Drawing for the job (mm, zero at the part's lowest x, y, z). A direction names the side the tool comes from. Give positions to 0.01 mm unless a question says otherwise; leave off trailing zeros. Loops run counter-clockwise (first coordinate to the right, second up) from the corner with the lowest first, then second, coordinate; pieces in that order, holes last. Notation, with made-up numbers: (36.25, -36) -> (43.25, -36) arc R16 ccw to (43.25, -6) -> close; hole circle Ø10 at (45, -6.5). An arc over 180 degrees is marked (long way). Use CSV: the item, a comma, the result in double quotes. Start each with the question number.
(1) Cut at D-D on z = 9. Write the cut outline in (x, y).
(2) Cut at B-B on y = 26.25. State how many separate pieces and enclosed holes the cut face has, then the cut area to 3 significant figures.
(3) 3-axis set-ups, long thin cutter, end or side, ignore diameter. For the marked faces 1, 2, 3, 4 and 5: which of +Z, -Z, +X, -X, +Y, -Y reach the whole face in a straight line?
(4) Drill centre lines: probe 1 along X at (y, z) = (26.8, 3); probe 2 along Z at (x, y) = (41.7, 19); probe 3 along Y at (x, z) = (7, 26.5). Where is each one in solid material? Low to high.
(5) Cut at C-C on x = 27. Write the cut outline in (y, z), then the cut area to 3 significant figures.
(6) Flat gauge pins, fed straight in: pin 1 (2.5 mm diameter, centred on y = 16.5, z = 8.5, fed in from -X); pin 2 (2 mm diameter, centred on x = 43, y = 10, fed in from -Z); pin 3 (2.5 mm diameter, centred on x = 37, y = 8, fed in from +Z). Where does each tip first touch, or does it go through?
(7) Cut at A-A on z = 15. Write the cut outline in (x, y).
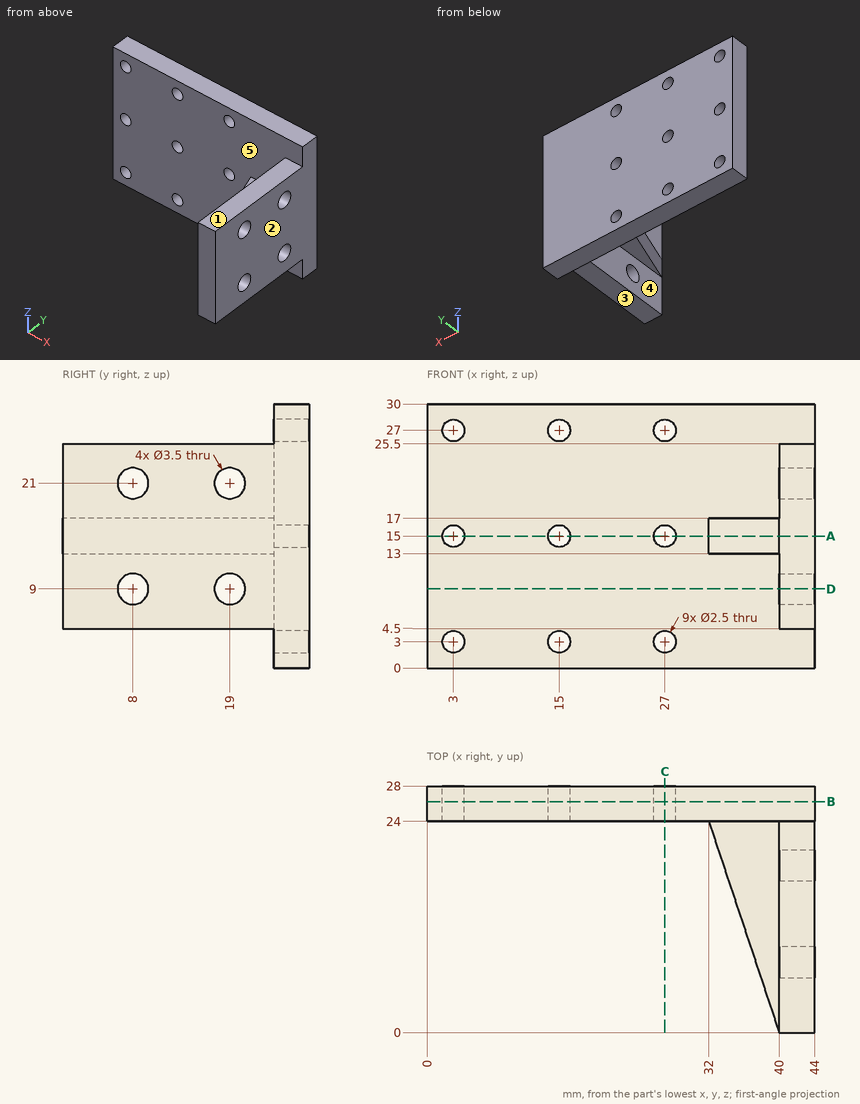
Check result:
1,outline,"(0, 24) -> (40, 24) -> (40, 20.75) -> (44, 20.75) -> (44, 28) -> (0, 28) -> close; (40, 0) -> (44, 0) -> (44, 6.25) -> (40, 6.25) -> close; (40, 9.75) -> (44, 9.75) -> (44, 17.25) -> (40, 17.25) -> close"
2,separate pieces,"1"
2,enclosed holes,"9"
2,area,"1,280 mm²"
3,face 1,"+Z, +X, -X, -Y"
3,face 2,"+Z, -Z, +X, +Y, -Y"
3,face 3,"-Z, +X, -X, -Y"
3,face 4,"-Z, -X, -Y"
3,face 5,"-X, -Y"
4,probe 1,"0 to 1.75, 4.25 to 13.75, 16.25 to 25.75, 28.25 to 44"
4,probe 2,"4.5 to 7.25, 10.75 to 19.25, 22.75 to 25.5"
4,probe 3,"24 to 28"
5,outline,"(24, 0) -> (28, 0) -> (28, 1.75) -> (24, 1.75) -> close; (24, 4.25) -> (28, 4.25) -> (28, 13.75) -> (24, 13.75) -> close; (24, 16.25) -> (28, 16.25) -> (28, 25.75) -> (24, 25.75) -> close; (24, 28.25) -> (28, 28.25) -> (28, 30) -> (24, 30) -> close"
5,area,"90.0 mm²"
6,pin 1,"x = 40"
6,pin 2,"z = 4.5"
6,pin 3,"z = 17"
7,outline,"(0, 24) -> (1.75, 24) -> (1.75, 28) -> (0, 28) -> close; (4.25, 24) -> (13.75, 24) -> (13.75, 28) -> (4.25, 28) -> close; (16.25, 24) -> (25.75, 24) -> (25.75, 28) -> (16.25, 28) -> close; (28.25, 24) -> (32, 24) -> (40, 0) -> (44, 0) -> (44, 28) -> (28.25, 28) -> close"
